For this review, take the finished solid that the model builds, in its own axes (mm). Face numbers are marked on the shaded views. Coordinates: 2 decimals unless noted, no trailing zeros. Order: outer loops, then holes, each group sorted by start corner. A loop starts at its lowest first (then second) coordinate and runs counter-clockwise, first axis right, second up. Notation, with made-up numbers: (59, 12) -> (72, 12) arc R25 cw to (72, 50) -> close; hole circle Ø2 at (-21.5, 83). An arc over 180 degrees is marked (long way). Return JSON: item names as keys, results as strings. Group by question number.
Item 1: Take a section at C-C (x = 0). Write out the cut boundary in (y, z), then the cut area to 3 significant figures.
Item 2: Take a section at A-A (x = 3.25). Write out the cut boundary in (y, z).
Item 3: Draft analysis for pull direction Z (two halves, no side actions). For the marked faces 1 and 2, state which applies: +Z half, -Z half, draft (parallel to the pull), parting line (faces both ways), or undercut.
Item 4: For line 1 along X through (y, z) = (44.05, 0); line 2 along X through (y, z) = (30, 0); line 3 along Z through (x, y) = (0, 43.7), list the stretches that pass through material, from the lowest coordinate up.
Item 5: Take a section at D-D (y = 41.5). Write out the cut boundary in (x, z), then the cut area to 3 significant figures.
Item 6: Take a section at B-B (z = -1.5). Write out the cut boundary in (x, y).
Item 7: Insertion check: pin 1 (6.5 mm diameter, centred on x = 0, z = 0, fed in from -Y) (3 decimals); pin 2 (5.5 mm diameter, centred on y = 25.5, z = 8.5, fed in from -X); pin 3 (3 mm diameter, centred on x = -4.5, y = 32, fed in from +Z); pin 4 (1.5 mm diameter, centred on x = -2, y = 18, fed in from -Z). Each pin has a flat end and moves straight along its axis. Give the tip position at first contact, or say it passes through.
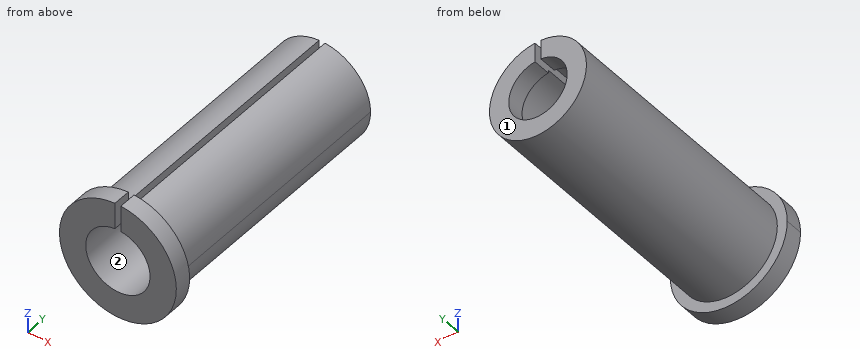
Autodesk Inventor part; units mm, degrees
ref_plane "YZ Plane" through (0, 0, 0) normal (1, 0, 0) x (0, 1, 0)
ref_plane "XZ Plane" through (0, 0, 0) normal (0, 1, 0) x (-1, 0, 0)
ref_plane "XY Plane" through (0, 0, 0) normal (0, 0, 1) x (1, 0, 0)
sketch "草圖1" plane through (0, 0, 0) normal (0, 1, 0) x (-1, 0, 0)
  circle A0 centre (0, 0) radius 10
  dimension "d0" = 20
extrude "擠出1" add sketch "草圖1" along normal blind 3
sketch "草圖2" plane through (0, 3, 0) normal (0, 1, 0) x (1, 0, 0)
  circle A0 centre (0, 0) radius 8.3
  circle A1 centre (0, 0) radius 5.5
  dimension "d3" = 16.6
  dimension "d4" = 11
extrude "擠出2" add sketch "草圖2" along normal blind 43 contours A0 | A1
sketch "草圖3" plane through (0, 0, 0) normal (0, -1, 0) x (1, 0, 0)
  circle A0 centre (0, 0) radius 5.5
  circle A1 centre (0, 0) radius 10
  dimension "d19" = 11
extrude "擠出3" cut sketch "草圖3" against normal blind 43 contours A0
sketch "草圖4" plane through (0, 46, 0) normal (0, 1, 0) x (1, 0, 0)
  point P0 (0, 0)
hole "孔1" at (0, 46, 0) direction (0, -1, 0) diameter 10 end through all
sketch "草圖5" plane through (0, 0, 0) normal (0, -1, 0) x (1, 0, 0)
  circle A0 centre (0, 0) radius 5
  circle A1 centre (0, 0) radius 10
  line L0 (0, 0) -> (0, 9.3404) construction
  line L1 (-0.5, 4.9749) -> (-0.5, 9.9875)
  line L2 (0.5, 4.9749) -> (0.5, 9.9875)
  dimension "d16" = 1
extrude "擠出4" cut sketch "草圖5" against normal through all contours A0 L1 A1 L2 picked at (0.0556, 6.6643)
properties part number "迫緊環"
Findings below:
{
 "1": {"outline": "(0, -10) -> (3, -10) -> (3, -8.3) -> (46, -8.3) -> (46, -5) -> (43, -5) -> (43, -5.5) -> (0, -5.5) -> close", "area": "135 mm2"},
 "2": {"outline": "(0, -9.46) -> (3, -9.46) -> (3, -7.64) -> (46, -7.64) -> (46, -3.8) -> (43, -3.8) -> (43, -4.44) -> (0, -4.44) -> close; (0, 4.44) -> (43, 4.44) -> (43, 3.8) -> (46, 3.8) -> (46, 7.64) -> (3, 7.64) -> (3, 9.46) -> (0, 9.46) -> close"},
 "3": {"face 1": "draft", "face 2": "undercut"},
 "4": {"line 1": "x = -8.3 to -5, 5 to 8.3", "line 2": "x = -8.3 to -5.5, 5.5 to 8.3", "line 3": "z = -8.3 to -5"},
 "5": {"outline": "(-0.5, 5.48) -> (-0.5, 8.28) arc R8.3 ccw (long way) to (0.5, 8.28) -> (0.5, 5.48) arc R5.5 cw (long way) to start", "area": "119 mm2"},
 "6": {"outline": "(-9.89, 0) -> (-5.29, 0) -> (-5.29, 43) -> (-4.77, 43) -> (-4.77, 46) -> (-8.16, 46) -> (-8.16, 3) -> (-9.89, 3) -> close; (4.77, 43) -> (5.29, 43) -> (5.29, 0) -> (9.89, 0) -> (9.89, 3) -> (8.16, 3) -> (8.16, 46) -> (4.77, 46) -> close"},
 "7": {"pin 1": "passes through", "pin 2": "stops at x = -5.99", "pin 3": "stops at z = 7.74", "pin 4": "stops at z = -8.21"}
}
